Geometry check sheet. Reference: the model listing, model coordinates, mm. A direction names the side the tool comes from. Give positions to 0.01 mm unless a question says otherwise; leave off trailing zeros. Loops run counter-clockwise (first coordinate to the right, second up) from the corner with the lowest first, then second, coordinate; pieces in that order, holes last. Notation, with made-up numbers: (16.25, 16.25) - (25.25, 16.25) arc R38 cw to (25.25, 55.25) - close; hole circle Ø3 at (36.5, -10). An arc over 180 degrees is marked (long way). Use a Markdown table: item, result. Add a question column.
1. Material ranges on L1, parallel to Y at x = -23.55, z = -9.5; L2, parallel to Z at x = -23.4, y = -40.75; L3, parallel to Z at x = -2, y = 33, recorded low to high.
2. Set-up check for faces 1 (the cylindrical face through (-0.31, 14.06, -0.49)), 2 (the cylindrical face through (-23.26, -43.06, -10.46)): record each of +Z, -Z, +X, -X, +Y, -Y from which the full face is reachable in a straight line by a thin tool's end or side.
3. Depth check by flat-ended pin: P1, Ø1.1, axis at x = -23, z = -8, coming from the -Y side; P2, Ø6, axis at x = -14.5, y = -19.5, coming from the -Z side; P3, Ø8, axis at y = 48.25, z = -9.5, coming from the -X side; P4, Ø1, axis at x = -2.5, z = -2.5, coming from the -Y side. Enter the tip coordinate at first touch or a pass-through.
4. Draft check along Y on faces 3 (the flat face through (0, 1, -1)), 4 (the cylindrical face through (-23.27, 53.39, -14.1)), 5 (the cylindrical face through (-15.35, 48.06, -0.49)). Enter one of: pulls with the +Y half, pulls with the -Y half, needs draft (parallel to the pull), parting line crosses it, or undercut.
5. Cross-section at C-C on y = -26. Enter the section's corners in (x, z).
6. Cross-section at B-B on y = 48.25. Enter the section's corners in (x, z), and give its area (3 significant figures).
7. Cross-section at A-A on z = -9.5. Enter the section's corners in (x, y).
from build123d import *

# Parameters (mm, degrees)
F1_DEPTH = 1
F2_DEPTH = 15
F4_D     = 5
F5_R     = 3
F6_DEPTH = 4


# Not quite as in the source:
# - a feature names something its author has since deleted; it is built from what else it names


with BuildPart() as f1:
    # F0 (on Top) → F1 (new body)
    with BuildSketch(Plane.XY):
        Polygon((24, 57.25), (-24, 57.25), (-24.0091441598, 54.25), (-22.5091511277, 54.2454279414), (-22.5091511277, 42.2454279414), (-22.5, -34.75), (-22.5, -46.75), (-24, -46.75), (-24, -57.25), (24, -57.25), align=None)
        with BuildLine():
            Line((13.9209458456, -22.2416133583), (-17.6390541544, -22.2416133583))
            ThreePointArc((-17.6390541544, -22.2416133583), (-19.8890541544, -19.9916133583), (-17.6390541544, -17.7416133583))
            Line((-17.6390541544, -17.7416133583), (13.9209458456, -17.7416133583))
            ThreePointArc((13.9209458456, -17.7416133583), (16.1709458456, -19.9916133583), (13.9209458456, -22.2416133583))
        make_face(mode=Mode.SUBTRACT)
        with BuildLine():
            Line((9.9809458456, -13.7416133583), (-17.6390541544, -13.7416133583))
            ThreePointArc((-17.6390541544, -13.7416133583), (-19.8890541544, -11.4916133583), (-17.6390541544, -9.2416133583))
            Line((-17.6390541544, -9.2416133583), (9.9809458456, -9.2416133583))
            ThreePointArc((9.9809458456, -9.2416133583), (12.2309458456, -11.4916133583), (9.9809458456, -13.7416133583))
        make_face(mode=Mode.SUBTRACT)
        with BuildLine():
            Line((6.0409458456, -5.2416133583), (-17.6390541544, -5.2416133583))
            ThreePointArc((-17.6390541544, -5.2416133583), (-19.8890541544, -2.9916133583), (-17.6390541544, -0.7416133583))
            Line((-17.6390541544, -0.7416133583), (6.0409458456, -0.7416133583))
            ThreePointArc((6.0409458456, -0.7416133583), (8.2909458456, -2.9916133583), (6.0409458456, -5.2416133583))
        make_face(mode=Mode.SUBTRACT)
        with BuildLine():
            Line((-19.9999999992, -31.5317022603), (-19.9999999992, -27.0317022603))
            Line((-19.9999999992, -27.0317022603), (16.0951670268, -27.0317022603))
            ThreePointArc((16.0951670268, -27.0317022603), (18.3824934665, -27.555243649), (19.9999999704, -29.25513498))
            Line((19.9999999704, -29.25513498), (19.991580365, -37.75513498))
            Line((19.991580365, -37.75513498), (6.1573753969, -37.7551350426))
            ThreePointArc((6.1573753969, -37.7551350426), (5.4441089744, -38.037790108), (4.9890264818, -38.6554816172))
            Line((4.9890264818, -38.6554816172), (4.9890264818, -40.6197120801))
            Line((4.9890264818, -40.6197120801), (19.9890264818, -40.6197120801))
            Line((19.9890264818, -40.6197120801), (20, -44.6197120801))
            Line((20, -44.6197120801), (0, -44.6197120801))
            Line((0, -44.6197120801), (0, -37.7900532508))
            ThreePointArc((0, -37.7900532508), (1.5958871284, -35.3350022858), (4.3312619815, -34.2900834468))
            Line((4.3312619815, -34.2900834468), (14.5000001306, -34.2900834468))
            Line((14.5000001306, -34.2900834468), (14.5000000048, -32.3122422563))
            ThreePointArc((14.5000000048, -32.3122422563), (14.2713851276, -31.7603171319), (13.7194600008, -31.5317022603))
            Line((13.7194600008, -31.5317022603), (-7.2499999992, -31.5317022603))
            Line((-7.2499999992, -31.5317022603), (-7.2499999992, -44.8960133593))
            Line((-7.2499999992, -44.8960133593), (-12.7499999992, -44.8960133593))
            Line((-12.7499999992, -44.8960133593), (-12.7499999992, -31.5317022603))
            Line((-12.7499999992, -31.5317022603), (-19.9999999992, -31.5317022603))
        make_face(mode=Mode.SUBTRACT)
        with BuildLine():
            Line((2.1009458456, 3.2583866417), (-17.6390541544, 3.2583866417))
            ThreePointArc((-17.6390541544, 3.2583866417), (-19.8890541544, 5.5083866417), (-17.6390541544, 7.7583866417))
            Line((-17.6390541544, 7.7583866417), (2.1009458456, 7.7583866417))
            ThreePointArc((2.1009458456, 7.7583866417), (4.3509458456, 5.5083866417), (2.1009458456, 3.2583866417))
        make_face(mode=Mode.SUBTRACT)
        with BuildLine():
            Line((-2.5590541544, 11.7583866417), (-17.6390541544, 11.7583866417))
            ThreePointArc((-17.6390541544, 11.7583866417), (-19.8890541544, 14.0083866417), (-17.6390541544, 16.2583866417))
            Line((-17.6390541544, 16.2583866417), (-2.5590541544, 16.2583866417))
            ThreePointArc((-2.5590541544, 16.2583866417), (-0.3090541544, 14.0083866417), (-2.5590541544, 11.7583866417))
        make_face(mode=Mode.SUBTRACT)
        with BuildLine():
            Line((-5.7790541544, 20.2583866417), (-17.6390541544, 20.2583866417))
            ThreePointArc((-17.6390541544, 20.2583866417), (-19.8890541544, 22.5083866417), (-17.6390541544, 24.7583866417))
            Line((-17.6390541544, 24.7583866417), (-5.7790541544, 24.7583866417))
            ThreePointArc((-5.7790541544, 24.7583866417), (-3.5290541544, 22.5083866417), (-5.7790541544, 20.2583866417))
        make_face(mode=Mode.SUBTRACT)
        with BuildLine():
            Line((-9.7190541544, 28.7583866417), (-17.6390541544, 28.7583866417))
            ThreePointArc((-17.6390541544, 28.7583866417), (-19.8890541544, 31.0083866417), (-17.6390541544, 33.2583866417))
            Line((-17.6390541544, 33.2583866417), (-9.7190541544, 33.2583866417))
            ThreePointArc((-9.7190541544, 33.2583866417), (-7.4690541544, 31.0083866417), (-9.7190541544, 28.7583866417))
        make_face(mode=Mode.SUBTRACT)
        with BuildLine():
            Line((-13.6590541544, 37.2583866417), (-17.6390541544, 37.2583866417))
            ThreePointArc((-17.6390541544, 37.2583866417), (-19.8890541544, 39.5083866417), (-17.6390541544, 41.7583866417))
            Line((-17.6390541544, 41.7583866417), (-13.6590541544, 41.7583866417))
            ThreePointArc((-13.6590541544, 41.7583866417), (-11.4090541544, 39.5083866417), (-13.6590541544, 37.2583866417))
        make_face(mode=Mode.SUBTRACT)
        with BuildLine():
            Line((-17.5990541544, 45.7583866417), (-17.6390541544, 45.7583866417))
            ThreePointArc((-17.6390541544, 45.7583866417), (-19.8890541544, 48.0083866417), (-17.6390541544, 50.2583866417))
            Line((-17.6390541544, 50.2583866417), (-17.5990541544, 50.2583866417))
            ThreePointArc((-17.5990541544, 50.2583866417), (-15.3490541544, 48.0083866417), (-17.5990541544, 45.7583866417))
        make_face(mode=Mode.SUBTRACT)
    extrude(amount=-F1_DEPTH)

    # F0 (on Top) → F2 (join)
    with BuildSketch(Plane.XY):
        Polygon((-22.5091511277, 54.2454279414), (-24.0091441598, 54.25), (-23.9357289877, 42.2454279414), (-22.5091511277, 42.2454279414), align=None)
        Polygon((-22.5, -34.75), (-23.997312058, -34.750000301), (-24, -46.75), (-22.5, -46.75), align=None)
    extrude(amount=-F2_DEPTH)

    # F4 (through all)
    with Locations(Plane.YZ):
        with Locations((-40.75, -9.5), (48.25, -9.5)):
            Hole(F4_D / 2)

    # F5
    f5_edges = [f1.edges().sort_by_distance(p)[0] for p in [
        (-23.22244, 42.245428, -15),
        (-23.259148, 54.247714, -15),
        (-23.248656, -34.75, -15),
        (-23.25, -46.75, -15),
    ]]
    fillet(f5_edges, radius=F5_R)

    # F0 (on Top) → F6 (join)
    with BuildSketch(Plane.XY):
        Polygon((-22.5091511277, 42.2454279414), (-23.9357289877, 42.2454279414), (-23.997312058, -34.750000301), (-22.5, -34.75), align=None)
    extrude(amount=-F6_DEPTH)


solid = f1.part
Values found:
| question | item | result |
|---|---|---|
| 1 | L1 | y = -46.75 to -43.25, -38.25 to -34.75, 42.25 to 45.75, 50.75 to 54.25 |
| 1 | L2 | z = -15 to -12, -7 to 0 |
| 1 | L3 | z = -1 to 0 |
| 2 | face 1 | +Z, -Z |
| 2 | face 2 | +X, -X |
| 3 | P1 | stops at y = -46.75 |
| 3 | P2 | stops at z = -1 |
| 3 | P3 | stops at x = -24 |
| 3 | P4 | passes through |
| 4 | face 3 | needs draft |
| 4 | face 4 | pulls with the +Y half |
| 4 | face 5 | undercut |
| 5 | outline | (-23.99, -4) - (-22.5, -4) - (-22.5, -1) - (24, -1) - (24, 0) - (-23.99, 0) - close |
| 6 | outline | (-23.97, -15) - (-22.51, -15) - (-22.51, -12) - (-23.97, -12) - close; (-23.97, -7) - (-22.51, -7) - (-22.51, -1) - (-19.88, -1) - (-19.88, 0) - (-23.97, 0) - close; (-15.36, -1) - (24, -1) - (24, 0) - (-15.36, 0) - close |
| 6 | area | 56.6 mm2 |
| 7 | outline | (-24.01, 54.25) - (-23.99, 50.75) - (-22.51, 50.75) - (-22.51, 54.25) - close; (-24, -46.75) - (-22.5, -46.75) - (-22.5, -43.25) - (-24, -43.25) - close; (-24, -38.25) - (-22.5, -38.25) - (-22.5, -34.75) - (-24, -34.75) - close; (-23.96, 45.75) - (-23.94, 42.25) - (-22.51, 42.25) - (-22.51, 45.75) - close |
